Input: part model. Units: mm. Frame: model coordinates. Face numbers are marked on the shaded views. A direction names the side the tool comes from. Give positions to 0.01 mm unless a question says otherwise; leave off trailing zeros. Order: outer loops, then holes, each group sorted by start corner. A loop starts at its lowest first (then second) coordinate and runs counter-clockwise, first axis right, second up. Notation, with made-up numbers: M 5.25,-0.5 L 31.25,-0.5 A23 cw 31.25,27.5 Z; hole C 51,-15 d2. An arc over 180 degrees is marked long. Use a Markdown table: item, result.
from build123d import *

# Parameters (mm, degrees)
BOSS_EXTRUDE1_DEPTH = 6.35


with BuildPart() as part:
    # Sketch1 → Boss-Extrude1 (new body)
    with BuildSketch(Plane.XY):
        with BuildLine():
            Line((-13.814468498, 55.753), (-0.512454363, 55.753))
            Line((-0.512454363, 55.753), (2.695531502, 55.756757116))
            Line((2.695531502, 55.756757116), (2.695531502, 43.818757116))
            Line((2.695531502, 43.818757116), (-3.654468498, 43.818757116))
            Line((-3.654468498, 43.818757116), (-3.654468498, 8.990868624))
            Line((-3.654468498, 8.990868624), (2.695531502, 8.990868624))
            Line((2.695531502, 8.990868624), (2.695531502, -2.512333634))
            ThreePointArc((2.695531502, -2.512333634), (30.527357476, 0.70923947), (57.236842715, 9.170472751))
            Line((57.236842715, 9.170472751), (54.325835419, 20.034499879))
            Line((54.325835419, 20.034499879), (66.593093413, 23.321501752))
            Line((66.593093413, 23.321501752), (63.30609154, 35.588759746))
            Line((63.30609154, 35.588759746), (60.796097964, 34.916208994))
            ThreePointArc((60.796097964, 34.916208994), (51.793653569, 30.444949555), (45.230580184, 22.831656326))
            Line((45.230580184, 22.831656326), (44.147031561, 20.904803413))
            ThreePointArc((44.147031561, 20.904803413), (41.295489117, 17.558815877), (37.391946488, 15.536618596))
            ThreePointArc((37.391946488, 15.536618596), (26.579212526, 12.858245248), (15.581150656, 11.088630994))
            ThreePointArc((15.581150656, 11.088630994), (14.379521981, 11.63871145), (14.317303994, 12.958798154))
            Line((14.317303994, 12.958798154), (32.704850479, 46.608917104))
            ThreePointArc((32.704850479, 46.608917104), (39.295996489, 54.397381198), (48.420216702, 58.963778482))
            Line((48.420216702, 58.963778482), (56.465172321, 61.119417843))
            Line((56.465172321, 61.119417843), (53.178170448, 73.386675837))
            Line((53.178170448, 73.386675837), (40.910912454, 70.099673965))
            Line((40.910912454, 70.099673965), (37.813569329, 81.659115874))
            ThreePointArc((37.813569329, 81.659115874), (23.44688739, 73.388727882), (7.621608316, 68.453))
            Line((7.621608316, 68.453), (-13.814468498, 68.453))
            ThreePointArc((-13.814468498, 68.453), (-26.514468498, 55.753), (-13.814468498, 43.053))
            Line((-13.814468498, 43.053), (-13.814468498, 55.753))
        make_face()
        with BuildLine():
            Line((24.264057522, 57.64700047), (11.43, 34.160040827))
            ThreePointArc((11.43, 34.160040827), (10.00126648, 33.538520613), (9.045531502, 34.769023557))
            Line((9.045531502, 34.769023557), (9.045531502, 54.745185852))
            ThreePointArc((9.045531502, 54.745185852), (9.335322516, 55.552706963), (10.072445431, 55.991704669))
            ThreePointArc((10.072445431, 55.991704669), (16.462813232, 57.486670752), (22.724329021, 59.452667759))
            ThreePointArc((22.724329021, 59.452667759), (24.115953694, 59.080021624), (24.264057522, 57.64700047))
        make_face(mode=Mode.SUBTRACT)
        Polygon((33.576896794, 54.82609289), (28.004554301, 57.871006542), (34.094381606, 69.015691526), (39.666724099, 65.970777874), align=None, mode=Mode.SUBTRACT)
        Polygon((18.649366076, 27.507973818), (13.077023583, 30.552887471), (6.987196278, 19.408202487), (12.559538771, 16.363288834), align=None, mode=Mode.SUBTRACT)
    extrude(amount=BOSS_EXTRUDE1_DEPTH)


solid = part.part
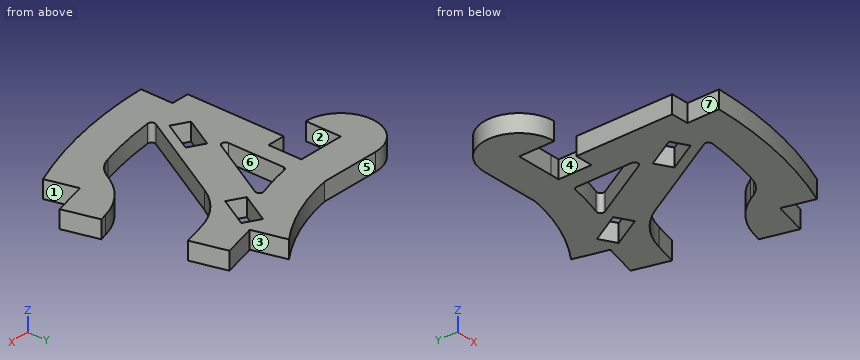
1) Cut plane B-B on y = 24.5. Return loops of the section in (x, z).
Response values:
| item | result |
|---|---|
| outline | M -3.65,0 L 9.77,0 L 9.77,6.35 L -3.65,6.35 Z; M 17.01,0 L 20.62,0 L 20.62,6.35 L 17.01,6.35 Z; M 46.26,0 L 66.28,0 L 66.28,6.35 L 46.26,6.35 Z |
2) Cut plane C-C on x = 31. Return loops of the section in (y, z), and give its area (3 significant figures).
Response values:
| item | result |
|---|---|
| outline | M 0.81,0 L 13.84,0 L 13.84,6.35 L 0.81,6.35 Z; M 43.49,0 L 56.23,0 L 56.23,6.35 L 43.49,6.35 Z; M 63.35,0 L 77.21,0 L 77.21,6.35 L 63.35,6.35 Z |
| area | 252 mm² |
3) Mould query, pull axis Y, two halves, no side actions, for the marked faces 1, 2, 3 and 4. Classes: released by +Y, released by -Y, zero draft, split by the parting line, or undercut.
Response values:
| item | result |
|---|---|
| face 1 | undercut |
| face 2 | zero draft |
| face 3 | released by +Y |
| face 4 | undercut |
4) Cut plane D-D on z = 5. State how many separate pieces and enclosed holes the cut face has, and give its area (3 significant figures).
Response values:
| item | result |
|---|---|
| separate pieces | 1 |
| enclosed holes | 3 |
| area | 3,120 mm² |
5) Material intervals for line 1 (Y direction, x = 31, z = 3); line 2 (Y direction, x = 31.5, z = 5.75); line 3 (X direction, y = 46.5, z = 3.5), sorted ascending. Write a range as from..to.
Response values:
| item | result |
|---|---|
| line 1 | y = 0.81..13.84, 43.49..56.23, 63.35..77.21 |
| line 2 | y = 0.92..13.96, 44.4..55.96, 64.27..77.5 |
| line 3 | x = -22.51..-13.81, 2.7..9.05, 18.17..32.65 |
6) Cut plane A-A on x = 1. Return loops of the section in (y, z), and give its area (3 significant figures).
Response values:
| item | result |
|---|---|
| outline | M 8.99,0 L 43.82,0 L 43.82,6.35 L 8.99,6.35 Z; M 55.75,0 L 68.45,0 L 68.45,6.35 L 55.75,6.35 Z |
| area | 302 mm² |
7) Reachability of the marked faces 5, 6 and 7 from +Z, -Z, +X, -X, +Y, -Y: full face, straight path, thin tool, end or side. Return the list, or none.
Response values:
| item | result |
|---|---|
| face 5 | +Z, -Z, -X, +Y |
| face 6 | +Z, -Z |
| face 7 | +Z, -Z, -X, -Y |
8) First-contact query: pin 1 Ø3 at (y, z) = (51.5, 4.5) entering from -X; pin 2 Ø1.9 at (x, z) = (-1, 3) entering from +Y; pin 3 Ø12 at (x, y) = (19.5, 39) entering from -Z; pin 4 Ø2 at (x, z) = (14, 3) entering from +Y. Flat tips, straight axial feed; report the tip coordinate or a pass-through.
Response values:
| item | result |
|---|---|
| pin 1 | stops at x = -26.21 |
| pin 2 | stops at y = 68.45 |
| pin 3 | stops at z = 0 |
| pin 4 | stops at y = 70.28 |
